Autodesk Inventor part; units mm, degrees
ref_plane "YZ Plane" through (0, 0, 0) normal (1, 0, 0) x (0, 1, 0)
ref_plane "XZ Plane" through (0, 0, 0) normal (0, 1, 0) x (-1, 0, 0)
ref_plane "XY Plane" through (0, 0, 0) normal (0, 0, 1) x (1, 0, 0)
sketch "Sketch1" plane through (0, 0, 0) normal (0, 0, 1) x (1, 0, 0)
  line L0 (0, 0) -> (97.5, 0)
  line L1 (97.5, 0) -> (97.5, 9)
  line L2 (97.5, 9) -> (0, 9)
  line L3 (0, 9) -> (0, 0)
  dimension "d2" = 97.5
  dimension "d3" = 9
extrude "Extrusion1" add sketch "Sketch1" along normal blind 5
sketch "Sketch2" plane through (0, 0, 5) normal (0, 0, 1) x (1, 0, 0)
  line L0 (0, 0) -> (97.5, 0)
  line L1 (97.5, 0) -> (97.5, 9)
  line L2 (0, 9) -> (0, 0)
  line L3 (2, 0) -> (32.5, 0)
  line L4 (32.5, 0) -> (32.5, 7)
  line L5 (32.5, 7) -> (2, 7)
  line L6 (2, 7) -> (2, 0)
  line L7 (33.5, 7) -> (64, 7)
  line L8 (64, 7) -> (64, 0)
  line L9 (64, 0) -> (33.5, 0)
  line L10 (33.5, 0) -> (33.5, 7)
  line L11 (65, 0) -> (95.5, 0)
  line L12 (95.5, 0) -> (95.5, 7)
  line L13 (95.5, 7) -> (65, 7)
  line L14 (65, 7) -> (65, 0)
  dimension "d4" = 7
  dimension "d5" = 30.5
  dimension "d6" = 2
  dimension "d7" = 2
  dimension "d8" = 30.5
  dimension "d9" = 30.5
  dimension "d10" = 1
extrude "Extrusion2" cut sketch "Sketch2" against normal blind 3
sketch "Sketch3" plane through (0, 0, 0) normal (-1, 0, 0) x (0, 0, 1)
  line L0 (0, 9) -> (0, 0)
  line L1 (0, 0) -> (5, 0)
  line L2 (0, 9) -> (2, 9)
  line L3 (2, 9) -> (2, 0)
  line L4 (2, 0) -> (0, 0)
  line L5 (0, 0) -> (0, 9)
  dimension "d13" = 2
extrude "Extrusion3" add sketch "Sketch3" along normal blind 7
sketch "Sketch5" plane through (97.5, 0, 0) normal (1, 0, 0) x (0, 0, -1)
  line L0 (0, 0) -> (-5, 0)
  line L1 (0, 9) -> (-2, 9)
  line L2 (-2, 9) -> (-2, 0)
  line L3 (-2, 0) -> (0, 0)
  line L4 (0, 0) -> (0, 9)
  dimension "d22" = 2
extrude "Extrusion5" add sketch "Sketch5" along normal blind 7
sketch "Sketch7" plane through (0, 0, 2) normal (0, 0, 1) x (1, 0, 0)
  line L0 (-7, 0) -> (-7, 9)
  line L1 (97.5, 0) -> (97.5, 9)
  line L2 (97.5, 0) -> (104.5, 0)
  line L3 (104.5, 9) -> (104.5, 0)
  line L4 (97.5, 9) -> (104.5, 9)
  point P0 (-3.5, 4.5)
  point P1 (101, 4.5)
  dimension "d31" = 3.5
  dimension "d32" = 4.5
  dimension "d33" = 3.5
hole "Hole1" at (-3.5, 4.5, 2) at (101, 4.5, 2) direction (0, 0, -1) diameter 3 end through all
fillet "Fillet1" radius 3 4 edges at (104.5, 0, 1) (104.5, 9, 1) (-7, 0, 1) (-7, 9, 1)
properties part number "base_corner" material "ABS Plastic"
CAD build for the part. Positions are in the model's coordinates, mm. A direction names the side the tool comes from. Give positions to 0.01 mm unless a question says otherwise; leave off trailing zeros. Write each loop counter-clockwise with the first axis right and the second up, starting at its lowest first coordinate (ties: lowest second). Pieces come first, ordered by that corner, then holes. Notation, with made-up numbers: M 78.5,88.25 L 121.5,88.25 A33 cw 121.5,121.25 Z; hole C -22,31 d7. An arc over 180 degrees is marked long. Return JSON: item names as keys, results as strings. Group by question number.
(1) Band-saw the part on B-B (z = 0.75). Give the cut face in (x, y), and give its area (3 significant figures).
(2) Mould opens along Y. For faces 4 (the face through (-2.6, 5.7, 1)), 5 (the face through (17, 7, 4)), 6 (the face through (2, 4, 4)) say: pulls with the +Y half, pulls with the -Y half, needs draft (parallel to the pull), parting line crosses it, or undercut.
(3) Band-saw the part on A-A (y = 4.5). Give the cut face in (x, z).
(4) Flat gauge pins, fed straight in: pin 1 Ø1 at (x, z) = (79, 3) entering from -Y; pin 2 Ø1.5 at (y, z) = (2.5, 4) entering from +X; pin 3 Ø2.5 at (y, z) = (2.5, 3.5) entering from -X. Where does each tip first touch, or does it go through?
(5) Band-saw the part on C-C (x = 42). Give the cut face in (y, z).
(6) Drill centre lines: L1, parallel to X at y = 4.5, z = 0.5; L2, parallel to X at y = 5.75, z = 4.5; L3, parallel to Y at x = 101, z = 1. Where is each one in solid material? Low to high. Write a range as [from, to].
(7) 3-axis set-ups, long thin cutter, end or side, ignore diameter. For faces 1 (the face through (0, 5, 3)), 2 (the face through (64, 4, 4)), 3 (the face through (-6.1, 8.14, 1.01)): which of +Z, -Z, +X, -X, +Y, -Y reach the whole face in a straight line?
Entries:
{
 "1": {"outline": "M -7,3 A3 ccw -4,0 L 101.5,0 A3 ccw 104.5,3 L 104.5,6 A3 ccw 101.5,9 L -4,9 A3 ccw -7,6 Z; hole C -3.5,4.5 d3; hole C 101,4.5 d3", "area": "982 mm^2"},
 "2": {"face 4": "undercut", "face 5": "pulls with the -Y half", "face 6": "needs draft"},
 "3": {"outline": "M -7,0 L -5,0 L -5,2 L -7,2 Z; M -2,0 L 99.5,0 L 99.5,2 L 97.5,2 L 97.5,5 L 95.5,5 L 95.5,2 L 65,2 L 65,5 L 64,5 L 64,2 L 33.5,2 L 33.5,5 L 32.5,5 L 32.5,2 L 2,2 L 2,5 L 0,5 L 0,2 L -2,2 Z; M 102.5,0 L 104.5,0 L 104.5,2 L 102.5,2 Z"},
 "4": {"pin 1": "stops at y = 7", "pin 2": "stops at x = 97.5", "pin 3": "stops at x = 0"},
 "5": {"outline": "M 0,0 L 9,0 L 9,5 L 7,5 L 7,2 L 0,2 Z"},
 "6": {"L1": "x = [-7, -5], [-2, 99.5], [102.5, 104.5]", "L2": "x = [0, 2], [32.5, 33.5], [64, 65], [95.5, 97.5]", "L3": "y = [0, 3], [6, 9]"},
 "7": {"face 1": "+Z, -X, +Y, -Y", "face 2": "+Z, -Y", "face 3": "+Z, -Z, -X, +Y"}
}
